from build123d import *

# Parameters (mm, degrees)
F1_DEPTH = 12
F2_W     = 14.1
F2_H     = 3.5
F3_DEPTH = 1.3
F4_R     = 1.5
F5_DEPTH = 3
F6_R     = 1.5
F7_DEPTH = 6.13
F8_R     = 1
F9_R     = 1


with BuildPart() as f1:
    # F0 (on Front) → F1 (new body)
    with BuildSketch(Plane.XZ):
        Polygon((-27.1, 0), (0, 0), (0, 6.13), (-11.3, 6.13), (-11.3, 4.63), (-10, 4.63), (-10, 3), (-24.1, 3), (-24.1, 4.63), (-22.8, 4.63), (-22.8, 6.13), (-27.1, 6.13), align=None)
    extrude(amount=F1_DEPTH)

    # F2 (on face) → F3 (cut)
    with BuildSketch(Plane.XY.offset(3)):
        with Locations((-17.05, -1.75)):
            Rectangle(F2_W, F2_H)
    extrude(amount=-F3_DEPTH, mode=Mode.SUBTRACT)

    # F4 (on face) → F5 (cut, through all)
    with BuildSketch(Plane.XY.offset(3)):
        with Locations((-17.05, -7.03)):
            Circle(F4_R)
    extrude(amount=-F5_DEPTH, mode=Mode.SUBTRACT)

    # F6 (on face) → F7 (cut, through all)
    with BuildSketch(Plane.XY.offset(6.13)):
        with Locations((-4.5, -7.03)):
            Circle(F6_R)
    extrude(amount=-F7_DEPTH, mode=Mode.SUBTRACT)

    # F8
    f8_edges = [f1.edges().sort_by_distance(p)[0] for p in [
        (-22.8, -6, 6.13),
        (-11.3, -6, 6.13),
        (-27.1, -6, 6.13),
        (0, -6, 6.13),
        (-17.05, -3.5, 3),
    ]]
    fillet(f8_edges, radius=F8_R)

    # F9
    f9_edges = [f1.edges().sort_by_distance(p)[0] for p in [
        (-24.1, -6, 4.63),
        (-10, -6, 4.63),
    ]]
    fillet(f9_edges, radius=F9_R)


solid = f1.part
Build history of the part. All positions in model axes, mm. A direction names the side the tool comes from. Round coordinates to 2 decimals unless told otherwise and drop trailing zeros. Loops run counter-clockwise (first coordinate to the right, second up) from the corner with the lowest first, then second, coordinate; pieces in that order, holes last. Notation, with made-up numbers: (70, 25.25) -> (128, 25.25) arc R26 cw to (128, 60.25) -> close; hole circle Ø1 at (55, -28.75). An arc over 180 degrees is marked (long way). Use CSV: the item, a comma, the result in double quotes. Start each with the question number.
Q1. Saw through at B-B on y = -7.03. Give the cut face in (x, z), and give its area (3 significant figures).
Q2. Saw through at C-C on x = -20. Give the cut face in (y, z).
Q3. Saw through at A-A on x = -17.05. Give the cut face in (y, z).
Q4. Mould opens along X. For faces 1 (the face through (-16.951, -3.801, 2.715)), 2 (the face through (-11, 0, 1)), 3 (the face through (0, -6, 3)), 4 (the face through (-26.815, -6.084, 5.829)) say: +X half, -X half, draft (parallel to the pull), parting line (faces both ways), or undercut.
Q5. Drill centre lines: L1, parallel to Y at x = -4.5, z = 2.75; L2, parallel to Y at x = -16, z = 2.75; L3, parallel to X at y = -10.75, z = 5. Where is each one in solid material? Low to high.
Q6. Flat gauge pins, fed straight in: pin 1 Ø1.5 at (x, y) = (-16, -10.5) entering from +Z; pin 2 Ø1 at (x, y) = (-20, -1) entering from +Z; pin 3 Ø6 at (x, y) = (-20, -9.5) entering from +Z. Where does each tip first touch, or does it go through?
Q7. Saw through at D-D on y = -1.5. Give the cut face in (x, z).
Q8. Which spindle directions (+Z, -Z, +X, -X, +Y, -Y) get a long thin tool onto all of the face, cutting with end or side? Do faces 5 (the face through (-24.1, -4.6, 3.3)), 6 (the face through (-23.799, -6.084, 4.345)), 7 (the face through (-23.101, -6.084, 5.845)). Say none if no direction does.
Solutions:
1,outline,"(-27.1, 0) -> (-18.55, 0) -> (-18.55, 3) -> (-24.1, 3) -> (-24.1, 3.63) arc R1 cw to (-23.1, 4.63) -> (-22.8, 4.63) -> (-22.8, 5.13) arc R1 ccw to (-23.8, 6.13) -> (-26.1, 6.13) arc R1 ccw to (-27.1, 5.13) -> close; (-15.55, 0) -> (-6, 0) -> (-6, 6.13) -> (-10.3, 6.13) arc R1 ccw to (-11.3, 5.13) -> (-11.3, 4.63) -> (-11, 4.63) arc R1 cw to (-10, 3.63) -> (-10, 3) -> (-15.55, 3) -> close; (-3, 0) -> (0, 0) -> (0, 5.13) arc R1 ccw to (-1, 6.13) -> (-3, 6.13) -> close"
1,area,"98.1 mm^2"
2,outline,"(-12, 0) -> (0, 0) -> (0, 1.7) -> (-3.5, 1.7) -> (-3.5, 2) arc R1 ccw to (-4.5, 3) -> (-12, 3) -> close"
3,outline,"(-12, 0) -> (-8.53, 0) -> (-8.53, 3) -> (-12, 3) -> close; (-5.53, 0) -> (0, 0) -> (0, 1.7) -> (-3.5, 1.7) -> (-3.5, 2) arc R1 ccw to (-4.5, 3) -> (-5.53, 3) -> close"
4,face 1,"undercut"
4,face 2,"draft"
4,face 3,"+X half"
4,face 4,"-X half"
5,L1,"y = -12 to -8.53, -5.53 to 0"
5,L2,"y = -12 to -8.1, -5.96 to -3.84"
5,L3,"x = -27.1 to -22.8, -11.3 to 0"
6,pin 1,"stops at z = 3"
6,pin 2,"stops at z = 1.7"
6,pin 3,"stops at z = 5.73"
7,outline,"(-27.1, 0) -> (0, 0) -> (0, 5.13) arc R1 ccw to (-1, 6.13) -> (-10.3, 6.13) arc R1 ccw to (-11.3, 5.13) -> (-11.3, 4.63) -> (-11, 4.63) arc R1 cw to (-10, 3.63) -> (-10, 1.7) -> (-24.1, 1.7) -> (-24.1, 3.63) arc R1 cw to (-23.1, 4.63) -> (-22.8, 4.63) -> (-22.8, 5.13) arc R1 ccw to (-23.8, 6.13) -> (-26.1, 6.13) arc R1 ccw to (-27.1, 5.13) -> close"
8,face 5,"+Y"
8,face 6,"+Y, -Y"
8,face 7,"+Z, +Y, -Y"
